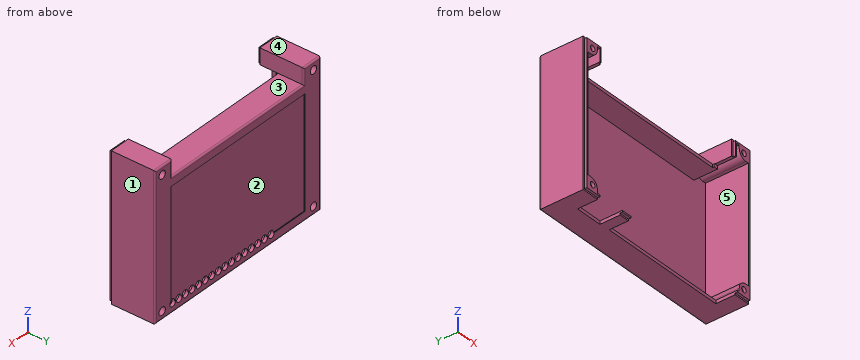
```python
from build123d import *

# Parameters (mm, degrees)
SKETCH_1_W             = 125.8
SKETCH_1_H             = 90
EXTRUDE_1_DEPTH        = 28.8
SKETCH_2_W             = 100
SKETCH_2_H             = 15
CUT_EXTRUDE_1_DEPTH    = 83.527874079
SHELL_1_T              = -2
SKETCH_3_W             = 106
SKETCH_3_H             = 3
CUT_EXTRUDE_2_DEPTH    = 12
EXTRUDE_2_DEPTH        = 26.8
SKETCH_5_R             = 1.75
CUT_EXTRUDE_3_DEPTH    = 83.527874079
SKETCH_6_R             = 2.4
CUT_EXTRUDE_4_DEPTH    = 27
SKETCH_7_W             = 101.8
SKETCH_7_H             = 69
CUT_EXTRUDE_5_DEPTH    = 0.5
FILLET_1_R             = 1
CUT_EXTRUDE_6_DEPTH    = 1.5
SKETCH_9_W             = 99
SKETCH_9_H             = 2
CUT_EXTRUDE_7_DEPTH    = 3
SKETCH_10_W            = 17
SKETCH_10_H            = 15
CUT_EXTRUDE_8_DEPTH    = 3
SKETCH_11_W            = 81
SKETCH_11_H            = 14.5
CUT_EXTRUDE_9_DEPTH    = 3
SKETCH_12_R            = 2.1
CUT_EXTRUDE_10_DEPTH   = 3
PATTERN_LINEAR_1_COUNT = 16
PATTERN_LINEAR_1_PITCH = 5


with BuildPart() as part:
    # Эскиз1 → Бобышка-Вытянуть1 (new body)
    with BuildSketch(Plane(origin=(0, 0, 0), x_dir=(1, 0, 0), z_dir=(0, 1, 0))):
        Rectangle(SKETCH_1_W, SKETCH_1_H)
    extrude(amount=EXTRUDE_1_DEPTH)

    # Эскиз2 → Вырез-Вытянуть1 (cut, through all)
    with BuildSketch(Plane(origin=(0, 28.8, 0), x_dir=(1, 0, 0), z_dir=(0, 1, 0))):
        with Locations((0, -42.5)):
            Rectangle(SKETCH_2_W, SKETCH_2_H)
    extrude(amount=-CUT_EXTRUDE_1_DEPTH, mode=Mode.SUBTRACT)

    # Оболочка1
    shell_1_openings = [part.faces().sort_by_distance(p)[0] for p in [
        (0, 0, -3.875217981),
    ]]
    offset(amount=SHELL_1_T, openings=shell_1_openings, kind=Kind.INTERSECTION)

    # Эскиз3 → Вырез-Вытянуть2 (cut)
    with BuildSketch(Plane.XZ):
        with Locations((0, 33.5)):
            Rectangle(SKETCH_3_W, SKETCH_3_H)
    extrude(amount=-CUT_EXTRUDE_2_DEPTH, mode=Mode.SUBTRACT)

    # Эскиз4 → Бобышка-Вытянуть2 (add)
    with BuildSketch(Plane.XZ.offset(-26.8)):
        with BuildLine():
            Line((-60.9, 43), (-53.9, 43))
            Line((-53.9, 43), (-53.9, 41))
            ThreePointArc((-53.9, 41), (-55.364466094, 37.464466094), (-58.9, 36))
            Line((-58.9, 36), (-60.9, 36))
            Line((-60.9, 36), (-60.9, 43))
        make_face()
        with BuildLine():
            Line((60.9, 43), (53.9, 43))
            Line((53.9, 43), (53.9, 41))
            ThreePointArc((53.9, 41), (55.364466094, 37.464466094), (58.9, 36))
            Line((58.9, 36), (60.9, 36))
            Line((60.9, 36), (60.9, 43))
        make_face()
        with BuildLine():
            Line((-60.9, -43), (-53.9, -43))
            Line((-53.9, -43), (-53.9, -41))
            ThreePointArc((-53.9, -41), (-55.364466094, -37.464466094), (-58.9, -36))
            Line((-58.9, -36), (-60.9, -36))
            Line((-60.9, -36), (-60.9, -43))
        make_face()
        with BuildLine():
            Line((60.9, -43), (53.9, -43))
            Line((53.9, -43), (53.9, -41))
            ThreePointArc((53.9, -41), (55.364466094, -37.464466094), (58.9, -36))
            Line((58.9, -36), (60.9, -36))
            Line((60.9, -36), (60.9, -43))
        make_face()
    extrude(amount=EXTRUDE_2_DEPTH)

    # Эскиз5 → Вырез-Вытянуть3 (cut, through all)
    with BuildSketch(Plane.XZ):
        with Locations(Location((-57.5, 40, 0), (0, 0, 270))):
            Circle(SKETCH_5_R)
        with Locations(Location((57.5, 40, 0), (0, 0, 270))):
            Circle(SKETCH_5_R)
        with Locations(Location((57.5, -40, 0), (0, 0, 270))):
            Circle(SKETCH_5_R)
        with Locations(Location((-57.5, -40, 0), (0, 0, 270))):
            Circle(SKETCH_5_R)
    extrude(amount=-CUT_EXTRUDE_3_DEPTH, mode=Mode.SUBTRACT)

    # Эскиз6 → Вырез-Вытянуть4 (cut)
    with BuildSketch(Plane(origin=(0, 28.8, 0), x_dir=(1, 0, 0), z_dir=(0, 1, 0))):
        with Locations(Location((-57.5, 40, 0), (0, 0, 270))):
            Circle(SKETCH_6_R)
        with Locations(Location((57.5, 40, 0), (0, 0, 270))):
            Circle(SKETCH_6_R)
        with Locations(Location((-57.5, -40, 0), (0, 0, 270))):
            Circle(SKETCH_6_R)
        with Locations(Location((57.5, -40, 0), (0, 0, 270))):
            Circle(SKETCH_6_R)
    extrude(amount=-CUT_EXTRUDE_4_DEPTH, mode=Mode.SUBTRACT)

    # Эскиз7 → Вырез-Вытянуть5 (cut)
    with BuildSketch(Plane(origin=(0, 28.8, 0), x_dir=(1, 0, 0), z_dir=(0, 1, 0))):
        with Locations((0, 5)):
            Rectangle(SKETCH_7_W, SKETCH_7_H)
    extrude(amount=-CUT_EXTRUDE_5_DEPTH, mode=Mode.SUBTRACT)

    # Скругление1
    fillet_1_edges = [part.edges().sort_by_distance(p)[0] for p in [
        (62.9, 28.8, 0),
        (0, 28.8, -45),
        (56.45, 28.8, 45),
        (50, 28.8, 40),
        (0, 28.8, 35),
        (-50, 28.8, 40),
        (-62.9, 28.8, 0),
        (-56.45, 28.8, 45),
    ]]
    fillet(fillet_1_edges, radius=FILLET_1_R)

    # Эскиз8 → Вырез-Вытянуть6 (cut)
    with BuildSketch(Plane.XZ):
        Polygon((-51, 32), (-51, 44), (-61.9, 44), (-61.9, -44), (61.9, -44), (61.9, 44), (51, 44), (51, 32), (49, 32), (49, 46), (63.9, 46), (63.9, -46), (-63.9, -46), (-63.9, 46), (-49, 46), (-49, 32), align=None)
    extrude(amount=-CUT_EXTRUDE_6_DEPTH, mode=Mode.SUBTRACT)

    # Эскиз9 → Вырез-Вытянуть7 (cut)
    with BuildSketch(Plane.XY.offset(35)):
        with Locations((0, 12)):
            Rectangle(SKETCH_9_W, SKETCH_9_H)
    extrude(amount=-CUT_EXTRUDE_7_DEPTH, mode=Mode.SUBTRACT)

    # Эскиз10 → Вырез-Вытянуть8 (cut)
    with BuildSketch(Plane(origin=(0, 0, -45), x_dir=(-1, 0, 0), z_dir=(0, 0, -1))):
        with Locations((43.4, 6.5)):
            Rectangle(SKETCH_10_W, SKETCH_10_H)
    extrude(amount=-CUT_EXTRUDE_8_DEPTH, mode=Mode.SUBTRACT)

    # Эскиз11 → Вырез-Вытянуть9 (cut)
    with BuildSketch(Plane(origin=(0, 0, -45), x_dir=(-1, 0, 0), z_dir=(0, 0, -1))):
        with Locations((-12, 6.25)):
            Rectangle(SKETCH_11_W, SKETCH_11_H)
    extrude(amount=-CUT_EXTRUDE_9_DEPTH, mode=Mode.SUBTRACT)

    # Эскиз12 → Вырез-Вытянуть10 (cut)
    with BuildSketch(Plane(origin=(0, 28.8, 0), x_dir=(1, 0, 0), z_dir=(0, 1, 0))):
        with Locations(Location((49.5, 39.5, 0), (0, 0, 270))):
            Circle(SKETCH_12_R)
    cut_extrude_10 = extrude(amount=-CUT_EXTRUDE_10_DEPTH, mode=Mode.SUBTRACT)

    # Линейный массив1: Вырез-Вытянуть10 ×16
    with Locations(*[(-i * PATTERN_LINEAR_1_PITCH, 0, 0) for i in range(1, PATTERN_LINEAR_1_COUNT)]):
        add(cut_extrude_10, mode=Mode.SUBTRACT)


solid = part.part
```
Check sheet for the modelled part. Datum: model origin and axes. Units: mm. Face numbers are marked on the shaded views. A direction names the side the tool comes from. Coordinates: 2 decimals unless noted, no trailing zeros. Order: outer loops, then holes, each group sorted by start corner. A loop starts at its lowest first (then second) coordinate and runs counter-clockwise, first axis right, second up. Notation, with made-up numbers: M 49.25,85.25 L 70.25,85.25 A9 cw 70.25,102.25 Z; hole C 57,78 d4. An arc over 180 degrees is marked long. One line per question, with ' | ' between items. Start each with the question number.
Item 1: Access from +Z, -Z, +X, -X, +Y, -Y to the whole of each face (thin tool, end or side, straight path). Record for the marked faces 4 and 5.
Item 2: Sectioned sample at C-C on x = 34.5. Record the cut outline in (y, z).
Item 3: Material ranges on line 1 (Z direction, x = 39.5, y = 27.9); line 2 (X direction, y = 10, z = 4.5); line 3 (Z direction, x = 32, y = 24.5), recorded low to high.
Item 4: Sectioned sample at D-D on z = 28. Record the cut outline in (x, y).
Item 5: Mould release check, pull along Z, two halves, no side actions. Record for the marked faces 1, 2 and 3: pulls with the +Z half, pulls with the -Z half, needs draft (parallel to the pull), parting line crosses it, or undercut.
Item 6: Sectioned sample at A-A on x = 57.5. Count the separate pieces of the cut face and the enclosed holes in it, and give its area (3 significant figures).
Item 7: Gauge pin test, flat ends, axial feed: P1, Ø6.5, axis at x = -25.5, z = -39.5, coming from the -Y side; P2, Ø4, axis at x = -57.5, z = -40, coming from the +Y side; P3, Ø0.6, axis at x = 22, y = 28.5, coming from the +Z side. Record the tip position at first contact, or that the pin passes through.
Answer below:
1) face 4: +Z, +X, -X, +Y, -Y | face 5: -Y
2) outline: M 13,33 L 26.8,33 L 26.8,-37.4 L 28.3,-37.4 L 28.3,29.5 L 28.8,29.5 L 28.8,34 A1 ccw 27.8,35 L 13,35 Z; M 13.5,-45 L 27.8,-45 A1 ccw 28.8,-44 L 28.8,-41.6 L 26.8,-41.6 L 26.8,-43 L 13.5,-43 Z
3) line 1: z = -44.99 to -41.6, -37.4 to 34.99 | line 2: x = -62.9 to -60.9, 60.9 to 62.9 | line 3: z = -45 to -43, 33 to 35
4) outline: M -62.9,1.5 L -61.9,1.5 L -61.9,0 L -60.9,0 L -60.9,26.8 L 60.9,26.8 L 60.9,0 L 61.9,0 L 61.9,1.5 L 62.9,1.5 L 62.9,27.8 A1 ccw 61.9,28.8 L 50.9,28.8 L 50.9,28.3 L -50.9,28.3 L -50.9,28.8 L -61.9,28.8 A1 ccw -62.9,27.8 Z
5) face 1: needs draft | face 2: undercut | face 3: pulls with the +Z half
6) separate pieces: 3 | enclosed holes: 0 | area: 376 mm^2
7) P1: stops at y = 26.8 | P2: stops at y = 1.8 | P3: stops at z = 34.92
